Can you work these out from the drawing? Everything is in mm from the part's minimum corner. A direction names the side the tool comes from. Round coordinates to 2 decimals unless told otherwise and drop trailing zeros. Write each loop counter-clockwise with the first axis right and the second up, starting at its lowest first coordinate (ties: lowest second). Pieces come first, ordered by that corner, then holes. Notation, with made-up numbers: (76.25, 51.25) -> (109.25, 51.25) arc R25 cw to (109.25, 76.25) -> close; hole circle Ø9 at (18.25, 12). An arc over 180 degrees is marked (long way). Answer as CSV lines item,"result".
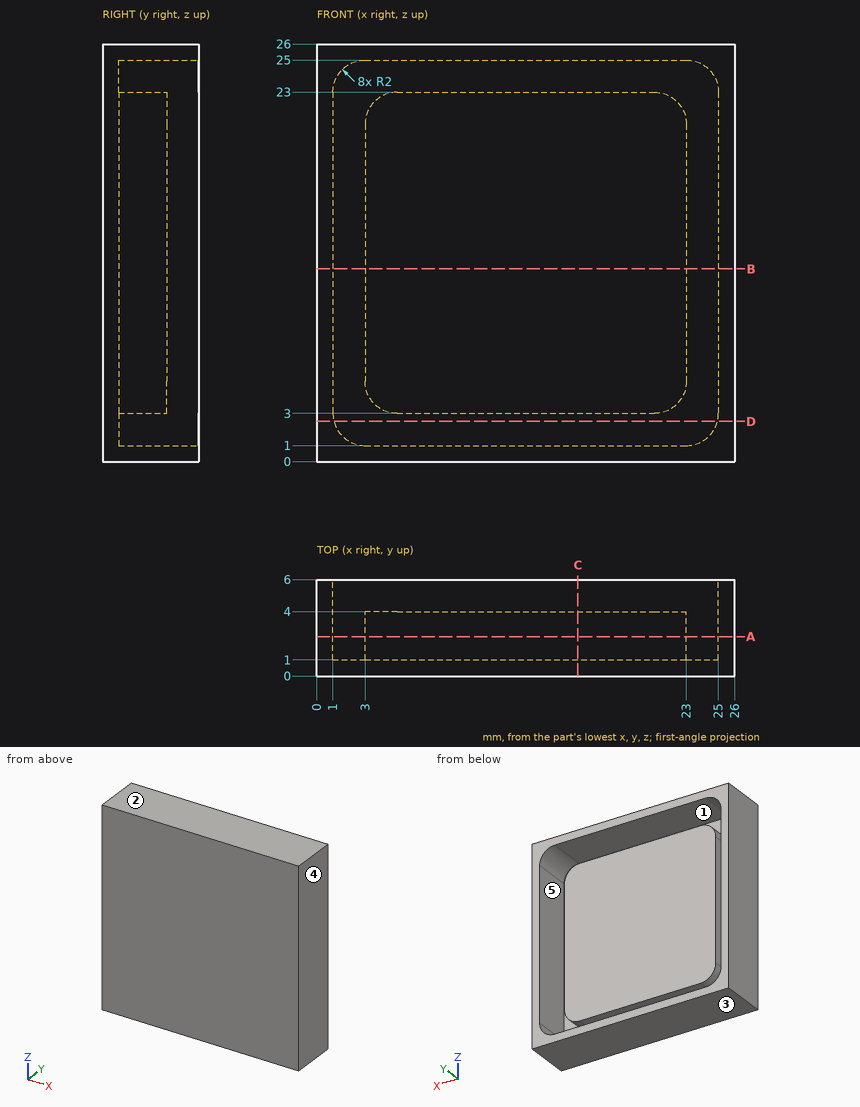
Item 1: I need wall thicknesses on L1, parallel to X at y = 3.55, z = 8.5; L2, parallel to Z at x = 11.5, y = 4.05. Which ranges of each line are inside material? Lowest first, please.
Results found:
L1,"x = 0 to 1, 3 to 23, 25 to 26"
L2,"z = 0 to 1, 25 to 26"
Item 2: Suppose I cut it at B-B, the plane z = 12. List the corners of the cut face in (x, y) for me.
Results found:
outline,"(0, 0) -> (26, 0) -> (26, 6) -> (25, 6) -> (25, 1) -> (23, 1) -> (23, 4) -> (3, 4) -> (3, 1) -> (1, 1) -> (1, 6) -> (0, 6) -> close"
Item 3: Suppose I cut it at C-C, the plane x = 16.25. List the corners of the cut face in (y, z) for me, then the cut area to 3 significant figures.
Results found:
outline,"(0, 0) -> (6, 0) -> (6, 1) -> (1, 1) -> (1, 3) -> (4, 3) -> (4, 23) -> (1, 23) -> (1, 25) -> (6, 25) -> (6, 26) -> (0, 26) -> close"
area,"96.0 mm²"
Item 4: If we mould it in two halves opening along X, with no side actions, what happens to the marked faces 3, 4 and 5? For each: pulls with the +X half, pulls with the -X half, needs draft (parallel to the pull), parting line crosses it, or undercut.
Results found:
face 3,"needs draft"
face 4,"pulls with the +X half"
face 5,"undercut"
Item 5: Suppose I cut it at D-D, the plane z = 2.5. List the corners of the cut face in (x, y) for me.
Results found:
outline,"(0, 0) -> (26, 0) -> (26, 6) -> (24.94, 6) -> (24.94, 1) -> (1.06, 1) -> (1.06, 6) -> (0, 6) -> close"
Item 6: Suppose I cut it at A-A, the plane y = 2.45. List the corners of the cut face in (x, z) for me, then the cut area to 3 significant figures.
Results found:
outline,"(0, 0) -> (26, 0) -> (26, 26) -> (0, 26) -> close; (3, 5) arc R2 ccw to (5, 3) -> (21, 3) arc R2 ccw to (23, 5) -> (23, 21) arc R2 ccw to (21, 23) -> (5, 23) arc R2 ccw to (3, 21) -> close; hole (1, 3) arc R2 ccw to (3, 1) -> (23, 1) arc R2 ccw to (25, 3) -> (25, 23) arc R2 ccw to (23, 25) -> (3, 25) arc R2 ccw to (1, 23) -> close"
area,"500 mm²"
Item 7: For the marked faces 1 and 2, which set-ups out of +Z, -Z, +X, -X, +Y, -Y let a thin tool reach every point of the face, with its end or its side?
Results found:
face 1,"+Y"
face 2,"+Z, +X, -X, +Y, -Y"
